Geometry check sheet. Reference: the model listing, model coordinates, mm. A direction names the side the tool comes from. Round coordinates to 2 decimals unless told otherwise and drop trailing zeros. Loops run counter-clockwise (first coordinate to the right, second up) from the corner with the lowest first, then second, coordinate; pieces in that order, holes last. Notation, with made-up numbers: M 24,42.5 L 63,42.5 A31 ccw 63,76.5 Z; hole C 43,28.25 d2. An arc over 180 degrees is marked long. Use one line per item in the form item = value. Start each with the question number.
1. Go/stop test with flat-tipped pins: pin 1 (6 mm diameter, centred on y = 811, z = 8, fed in from +X); pin 2 (2 mm diameter, centred on x = 13.5, y = 240, fed in from +Z); pin 3 (5 mm diameter, centred on x = -4, z = 10.5, fed in from +Y). Record where each tip stops, or that it passes through.
2. Cross-section at B-B (y = 356). Record the boundary of the cut face in (x, z).
3. Set-up check for faces 1 (the flat face through (2, 613, -15)), 2 (the flat face through (-18, 605, 20)): record each of +Z, -Z, +X, -X, +Y, -Y from which the full face is reachable in a straight line by a thin tool's end or side.
4. Material ranges on line 1 (X direction, y = 2, z = 0); line 2 (Y direction, x = 10, z = 9); line 3 (Z direction, x = 6, y = 562.5), recorded low to high.
5. Cross-section at A-A (z = 13). Record the boundary of the cut face in (x, y), then the cut area to 3 significant figures.
```python
from build123d import *

# Parameters (mm, degrees)
SKETCH_1_W          = 40
SKETCH_1_H          = 40
EXTRUDE_1_DEPTH     = 5
SKETCH_2_R          = 4.05
CUT_EXTRUDE_1_DEPTH = 5
EXTRUDE_2_DEPTH     = 600


with BuildPart() as part:
    # 草图1 → 凸台-拉伸1 (new body)
    with BuildSketch(Plane(origin=(0, 0, 0), x_dir=(1, 0, 0), z_dir=(0, 1, 0))):
        Rectangle(SKETCH_1_W, SKETCH_1_H)
    extrude(amount=EXTRUDE_1_DEPTH)

    # 草图2 → 切除-拉伸1 (cut)
    with BuildSketch(Plane(origin=(0, 5, 0), x_dir=(1, 0, 0), z_dir=(0, 1, 0))):
        with Locations(Location((0, 0, 0), (0, 0, 270))):
            Circle(SKETCH_2_R)
    extrude(amount=-CUT_EXTRUDE_1_DEPTH, mode=Mode.SUBTRACT)

    # 草图3 → 凸台-拉伸2 (add)
    with BuildSketch(Plane(origin=(0, 5, 0), x_dir=(1, 0, 0), z_dir=(0, 1, 0))):
        Polygon((-20, 20), (-20, -20), (-15, -20), (-15, 15), (20, 15), (20, 20), align=None)
    extrude_2 = extrude(amount=EXTRUDE_2_DEPTH)

    # 镜向1: 凸台-拉伸2 across plane
    add(extrude_2.mirror(Plane.ZX.offset(605)))


solid = part.part
```
Reported:
q1.pin_1 = -15
q1.pin_2 = -15
q1.pin_3 = 5
q2.outline = M -20,-20 L 20,-20 L 20,-15 L -15,-15 L -15,20 L -20,20 Z
q3.face_1 = +Z, +X, +Y
q3.face_2 = +Z, +X, -X, +Y, -Y
q4.line_1 = -20 to -4.05, 4.05 to 20
q4.line_2 = 0 to 5
q4.line_3 = -20 to -15
q5.outline = M -20,0 L 20,0 L 20,5 L -15,5 L -15,1205 L -20,1205 Z
q5.area = 6,200 mm²
